Geometry: final body of the model. Coordinates: model frame, mm. A direction names the side the tool comes from. Give positions to 0.01 mm unless a question says otherwise; leave off trailing zeros. Write each loop counter-clockwise with the first axis right and the second up, starting at its lowest first coordinate (ties: lowest second). Pieces come first, ordered by that corner, then holes.
```python
from build123d import *

# Parameters (mm, degrees)
Y_KSEKLIK_EKSTR_ZYON2_DEPTH = 10
IZIM3_W                     = 10
IZIM3_H                     = 40
Y_KSEKLIK_EKSTR_ZYON3_DEPTH = 10
IZIM4_W                     = 10
IZIM4_H                     = 133.89
Y_KSEKLIK_EKSTR_ZYON4_DEPTH = 10
IZIM6_W                     = 10
IZIM6_H                     = 50
Y_KSEKLIK_EKSTR_ZYON5_DEPTH = 10
IZIM7_W                     = 10
IZIM7_H                     = 142
Y_KSEKLIK_EKSTR_ZYON6_DEPTH = 10
IZIM8_R                     = 1.5
KES_EKSTR_ZYON1_DEPTH       = 35
IZIM9_R                     = 1.5
KES_EKSTR_ZYON2_DEPTH       = 374
IZIM12_R                    = 51
KES_EKSTR_ZYON4_DEPTH       = 338
Y_KSEKLIK_EKSTR_ZYON7_DEPTH = 5
Y_KSEKLIK_EKSTR_ZYON8_DEPTH = 5
IZIM21_W                    = 13.275114184
IZIM21_H                    = 150
KES_EKSTR_ZYON5_DEPTH       = 2.5
IZIM22_W                    = 15.470706389
IZIM22_H                    = 150
KES_EKSTR_ZYON6_DEPTH       = 2.5
IZIM23_R                    = 1.5
KES_EKSTR_ZYON7_DEPTH       = 242


with BuildPart() as part:
    # Çizim1 → Yükseklik-Ekstrüzyon2 (new body)
    with BuildSketch(Plane.XY):
        Polygon((-160, 89.142135624), (-90.502525317, 158.639610307), (90.502525317, 158.639610307), (160, 89.142135624), (160, -89.142135624), (90.502525317, -158.639610307), (-90.502525317, -158.639610307), (-160, -89.142135624), align=None)
        Polygon((-150, 85), (-150, -85), (-86.360389693, -148.639610307), (86.360389693, -148.639610307), (150, -85), (150, 85), (86.360389693, 148.639610307), (-86.360389693, 148.639610307), align=None, mode=Mode.SUBTRACT)
    extrude(amount=Y_KSEKLIK_EKSTR_ZYON2_DEPTH)

    # Çizim3 → Yükseklik-Ekstrüzyon3 (add)
    with BuildSketch(Plane(origin=(0, -123.89, 0), x_dir=(1, 0, 0), z_dir=(0, 1, 0))):
        with Locations((-112.926952731, -30)):
            Rectangle(IZIM3_W, IZIM3_H)
    y_kseklik_ekstr_zyon3 = extrude(amount=-Y_KSEKLIK_EKSTR_ZYON3_DEPTH)

    # Çizim4 → Yükseklik-Ekstrüzyon4 (add)
    with BuildSketch(Plane.XY.offset(50)):
        with Locations((-112.926952731, -66.945)):
            Rectangle(IZIM4_W, IZIM4_H)
    y_kseklik_ekstr_zyon4 = extrude(amount=Y_KSEKLIK_EKSTR_ZYON4_DEPTH)

    # Çizim6 → Yükseklik-Ekstrüzyon5 (add)
    with BuildSketch(Plane(origin=(0, -142, 0), x_dir=(1, 0, 0), z_dir=(0, 1, 0))):
        with Locations((103.073047269, -35)):
            Rectangle(IZIM6_W, IZIM6_H)
    y_kseklik_ekstr_zyon5 = extrude(amount=Y_KSEKLIK_EKSTR_ZYON5_DEPTH)

    # Çizim7 → Yükseklik-Ekstrüzyon6 (add)
    with BuildSketch(Plane.XY.offset(50)):
        with Locations((103.073047269, -71)):
            Rectangle(IZIM7_W, IZIM7_H)
    y_kseklik_ekstr_zyon6 = extrude(amount=Y_KSEKLIK_EKSTR_ZYON6_DEPTH)

    # Aynalama1: Yükseklik-Ekstrüzyon3, Yükseklik-Ekstrüzyon4, Yükseklik-Ekstrüzyon5, Yükseklik-Ekstrüzyon6 across plane
    add(y_kseklik_ekstr_zyon3.mirror(Plane.ZX))
    add(y_kseklik_ekstr_zyon4.mirror(Plane.ZX))
    add(y_kseklik_ekstr_zyon5.mirror(Plane.ZX))
    add(y_kseklik_ekstr_zyon6.mirror(Plane.ZX))

    # Çizim8 → Kes-Ekstrüzyon1 (cut)
    with BuildSketch(Plane.XY.offset(10)):
        with Locations((125, 117.071067812)):
            Circle(IZIM8_R)
        with Locations((119.343145751, 122.727922061)):
            Circle(IZIM8_R)
        with Locations((119.343145751, -122.727922061)):
            Circle(IZIM8_R)
        with Locations((125, -117.071067812)):
            Circle(IZIM8_R)
        with Locations((-140.343145751, 101.727922061)):
            Circle(IZIM8_R)
        with Locations((-146, 96.071067812)):
            Circle(IZIM8_R)
        with Locations((-140.343145751, -101.727922061)):
            Circle(IZIM8_R)
        with Locations((-146, -96.071067812)):
            Circle(IZIM8_R)
        with Locations((-155, 0)):
            Circle(IZIM8_R)
    extrude(amount=-KES_EKSTR_ZYON1_DEPTH, mode=Mode.SUBTRACT)

    # Çizim9 → Kes-Ekstrüzyon2 (cut)
    with BuildSketch(Plane(origin=(0, -142, 0), x_dir=(1, 0, 0), z_dir=(0, 1, 0))):
        with Locations(Location((-4, -4.992750184, 0), (0, 0, 90))):
            Circle(IZIM9_R)
        with Locations(Location((4, -4.992750184, 0), (0, 0, 90))):
            Circle(IZIM9_R)
    extrude(amount=KES_EKSTR_ZYON2_DEPTH, mode=Mode.SUBTRACT)

    # Çizim12 → Kes-Ekstrüzyon4 (cut, symmetric)
    with BuildSketch(Plane(origin=(-112.93, 0, 0), x_dir=(0, 0, -1), z_dir=(1, 0, 0))):
        with Locations((-69.443489697, 0)):
            Circle(IZIM12_R)
    extrude(amount=KES_EKSTR_ZYON4_DEPTH, both=True, mode=Mode.SUBTRACT)

    # Çizim19 → Yükseklik-Ekstrüzyon7 (add, symmetric)
    with BuildSketch(Plane(origin=(-112.93, 0, 0), x_dir=(0, 0, -1), z_dir=(1, 0, 0))):
        with BuildLine():
            Line((-50, -62.023791471), (-50, -47.148178209))
            ThreePointArc((-50, -47.148178209), (-18.443489697, 0), (-50, 47.148178209))
            Line((-50, 47.148178209), (-50, 62.023791471))
            ThreePointArc((-50, 62.023791471), (-4.443489697, 0), (-50, -62.023791471))
        make_face()
    extrude(amount=Y_KSEKLIK_EKSTR_ZYON7_DEPTH, both=True)

    # Çizim20 → Yükseklik-Ekstrüzyon8 (add, symmetric)
    with BuildSketch(Plane(origin=(103.07, 0, 0), x_dir=(0, 0, -1), z_dir=(1, 0, 0))):
        with BuildLine():
            Line((-50, -47.148178209), (-50, -62.023791471))
            ThreePointArc((-50, -62.023791471), (-4.443489697, 0), (-50, 62.023791471))
            Line((-50, 62.023791471), (-50, 47.148178209))
            ThreePointArc((-50, 47.148178209), (-18.443489697, 0), (-50, -47.148178209))
        make_face()
    extrude(amount=Y_KSEKLIK_EKSTR_ZYON8_DEPTH, both=True)

    # Çizim21 → Kes-Ekstrüzyon5 (cut, symmetric)
    with BuildSketch(Plane(origin=(-112.93, 0, 0), x_dir=(0, 0, -1), z_dir=(1, 0, 0))):
        with Locations((-56.637557092, 0)):
            Rectangle(IZIM21_W, IZIM21_H)
    extrude(amount=KES_EKSTR_ZYON5_DEPTH, both=True, mode=Mode.SUBTRACT)

    # Çizim22 → Kes-Ekstrüzyon6 (cut, symmetric)
    with BuildSketch(Plane(origin=(103.07, 0, 0), x_dir=(0, 0, -1), z_dir=(1, 0, 0))):
        with Locations((-57.735353195, 0)):
            Rectangle(IZIM22_W, IZIM22_H)
    extrude(amount=KES_EKSTR_ZYON6_DEPTH, both=True, mode=Mode.SUBTRACT)

    # Çizim23 → Kes-Ekstrüzyon7 (cut, symmetric)
    with BuildSketch(Plane(origin=(-112.93, 0, 0), x_dir=(0, 0, -1), z_dir=(1, 0, 0))):
        with Locations((-56.443489697, 60)):
            Circle(IZIM23_R)
        with Locations((-56.443489697, -60)):
            Circle(IZIM23_R)
    extrude(amount=KES_EKSTR_ZYON7_DEPTH, both=True, mode=Mode.SUBTRACT)


solid = part.part
```
Item 1: Section A-A, the plane x = 81.5. Return the cut outline in (y, z), plus the area to 3 significant figures.
Found:
outline: (-158.64, 0) - (-148.64, 0) - (-148.64, 10) - (-158.64, 10) - close; (148.64, 0) - (158.64, 0) - (158.64, 10) - (148.64, 10) - close
area: 200 mm2
Item 2: Pull-direction query (X, two-part tool) for faces 1 (the face through (-113, -123.89, 30)), 2 (the face through (-124.76, -124.38, 4.93)), 3 (the face through (105.57, 61, 55)), 4 (the face through (-150, 1, 5)); classes: +X half, -X half, draft (parallel to the pull), parting line (faces both ways), or undercut.
Found:
face 1: draft
face 2: -X half
face 3: undercut
face 4: undercut
Item 3: Section C-C, the plane z = 38. State how many separate pieces and enclosed holes the cut face has, plus the area to 3 significant figures.
Found:
separate pieces: 8
enclosed holes: 0
area: 1,070 mm2
Item 4: Pin query (flat end, axial travel): pin 1 Ø2.5 at (x, y) = (-155, 0) entering from -Z; pin 2 Ø3 at (x, z) = (103, 20.5) entering from -Y; pin 3 Ø5.5 at (x, z) = (-112, 57.5) entering from -Y; pin 4 Ø4 at (x, y) = (-146, 96.07) entering from +Z. Return the tip coordinate at first contact, or that it passes through.
Found:
pin 1: passes through
pin 2: stops at y = -142
pin 3: stops at y = -133.89
pin 4: stops at z = 10
Item 5: Reachability of faces 5 (the face through (-107.927, -103, 52)), 6 (the face through (150, -1, 5)), 7 (the face through (100.57, 61, 55)) from +Z, -Z, +X, -X, +Y, -Y: full face, straight path, thin tool, end or side. Return the list, or none.
Found:
face 5: +Z, +Y, -Y
face 6: +Z, -Z
face 7: +Z
Item 6: Section B-B, the plane y = -39.5. Return the cut outline in (x, z), plus the area to 3 significant figures.
Found:
outline: (-160, 0) - (-150, 0) - (-150, 10) - (-160, 10) - close; (-117.93, 17.82) - (-107.93, 17.82) - (-107.93, 37.18) - (-117.93, 37.18) - close; (98.07, 17.82) - (108.07, 17.82) - (108.07, 37.18) - (98.07, 37.18) - close; (150, 0) - (160, 0) - (160, 10) - (150, 10) - close
area: 587 mm2
Item 7: Section D-D, the plane y = 20. Return the cut outline in (x, z).
Found:
outline: (-160, 0) - (-150, 0) - (-150, 10) - (-160, 10) - close; (-117.93, 7.6) - (-107.93, 7.6) - (-107.93, 22.53) - (-117.93, 22.53) - close; (98.07, 7.6) - (108.07, 7.6) - (108.07, 22.53) - (98.07, 22.53) - close; (150, 0) - (160, 0) - (160, 10) - (150, 10) - close
Item 8: Line query: L1, parallel to X at y = 61.5, z = 50.5; L2, parallel to X at y = 82, z = 3; L3, parallel to Y at x = 35.5, z = 4.5. Output: solid intervals per line, ascending.
Found:
L1: x = -117.93 to -115.43, -110.43 to -107.93, 98.07 to 100.57, 105.57 to 108.07
L2: x = -160 to -150, 150 to 160
L3: y = -158.64 to -148.64, 148.64 to 158.64
